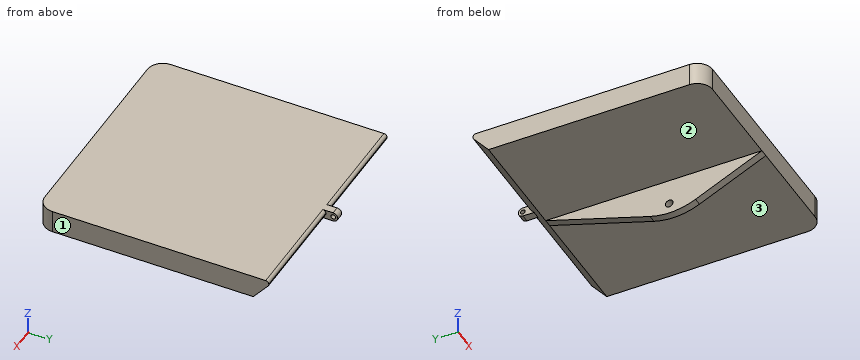
```python
from build123d import *

# Parameters (mm, degrees)
F0_W     = 150
F0_H     = 15
F1_DEPTH = 75
F2_SIZE2 = 10.0691955741
F2_SIZE  = 12
F3_R     = 2
F4_R     = 2.5
F5_DEPTH = 2.5
F6_R     = 1.5
F7_DEPTH = 2.5
F8_R     = 10


with BuildPart() as f1:
    # F0 (on Right) → F1 (new body, symmetric)
    with BuildSketch(Plane.YZ):
        with Locations((15, 24.5)):
            Rectangle(F0_W, F0_H)
    extrude(amount=F1_DEPTH, both=True)

    # F2
    f2_edges = [f1.edges().sort_by_distance(p)[0] for p in [
        (0, 90, 17),
    ]]
    f2_side = f1.faces().sort_by_distance((0, 90, 24.5))[0]
    chamfer(f2_edges, length=F2_SIZE, length2=F2_SIZE2, reference=f2_side)

    # F3
    f3_edges = [f1.edges().sort_by_distance(p)[0] for p in [
        (0, 90, 32),
        (0, 90, 29),
    ]]
    fillet(f3_edges, radius=F3_R)

    # F4 (on Right) → F5 (join, symmetric)
    with BuildSketch(Plane.YZ):
        with BuildLine():
            Line((79.9308044259, 17), (-60, 17))
            Line((-60, 17), (-17.0128849215, -3.2016815445))
            ThreePointArc((-17.0128849215, -3.2016815445), (-2.4781851934, -6.9231586695), (12.4051748829, -5.0277745355))
            Line((12.4051748829, -5.0277745355), (79.9308044259, 17))
        make_face()
        Circle(F4_R, mode=Mode.SUBTRACT)
    extrude(amount=F5_DEPTH, both=True)

    # F6 (on Right) → F7 (join, symmetric)
    with BuildSketch(Plane.YZ):
        with BuildLine():
            Line((94.6649461985, 32), (84.0871334076, 32))
            Line((84.0871334076, 32), (84.0871334076, 26))
            Line((84.0871334076, 26), (94.6649461985, 26))
            ThreePointArc((94.6649461985, 26), (97.6649461985, 29), (94.6649461985, 32))
        make_face()
        with Locations((94.6649461985, 29)):
            Circle(F6_R, mode=Mode.SUBTRACT)
    extrude(amount=F7_DEPTH, both=True)

    # F8
    f8_edges = [f1.edges().sort_by_distance(p)[0] for p in [
        (75, -60, 24.5),
        (-75, -60, 24.5),
    ]]
    fillet(f8_edges, radius=F8_R)


solid = f1.part
```
The listing builds one solid part. Answer for the finished solid, in the listing's coordinates (mm). Face numbers are marked on the shaded views. A direction names the side the tool comes from. Give positions to 0.01 mm unless a question says otherwise; leave off trailing zeros. Order: outer loops, then holes, each group sorted by start corner. A loop starts at its lowest first (then second) coordinate and runs counter-clockwise, first axis right, second up. Notation, with made-up numbers: M 88,-27.5 L 119,-27.5 A19 ccw 119,-3.5 Z; hole C 56.5,-11.75 d6. An arc over 180 degrees is marked long. Put each result on its own line as item: value. Start each with the question number.
Item 1: The part is cut by section D-D, the plane x = 37.5. Determine the outline of the cut face in (y, z).
Item 2: Which of the six approach directions +Z, -Z, +X, -X, +Y, -Y give full straight-line access (tool end or side, diameter ignored) to the marked faces 1, 2 and 3?
Item 3: The part is cut by section B-B, the plane y = 0. Determine the outline of the cut face in (x, z), and give its area (4 significant figures).
Item 4: Find the intervals of material crossed by line 1 along Z through (x, y) = (1, 0); line 2 along Z through (x, y) = (24, -2.5); line 3 along X through (y, z) = (-43.5, 10.5), in increasing order.
Item 5: The part is cut by section C-C, the plane z = 0. Determine the outline of the cut face in (x, y).
Item 6: The part is cut by section A-A, the plane x = 0.5. Determine the outline of the cut face in (y, z), and give its area (3 significant figures).
Item 7: Flat-ended cylindrical pins translate along their axes: P1, Ø10, axis at y = -39, z = 3, coming from the -X side; P2, Ø10, axis at x = 35.5, y = 8, coming from the -Z side; P3, Ø3.5, axis at y = 94.66, z = 29, coming from the +X side. Find the tip coordinate at first contact, or state that the pin passes through.
Answer key:
1. outline: M -60,17 L 79.93,17 L 89.53,28.44 A2 ccw 90,29.73 L 90,30 A2 ccw 88,32 L -60,32 Z
2. face 1: +Z, -Z, +X, +Y, -Y
2. face 2: -Z, -X, +Y, -Y
2. face 3: -Z, +X, +Y, -Y
3. outline: M -75,17 L -2.5,17 L -2.5,2.5 L 2.5,2.5 L 2.5,17 L 75,17 L 75,32 L -75,32 Z; M -2.5,-7 L 2.5,-7 L 2.5,-2.5 L -2.5,-2.5 Z
3. area: 2,345 mm²
4. line 1: z = -7 to -2.5, 2.5 to 32
4. line 2: z = 17 to 32
4. line 3: x = -2.5 to 2.5
5. outline: M -2.5,-23.83 L 2.5,-23.83 L 2.5,-2.5 L -2.5,-2.5 Z; M -2.5,2.5 L 2.5,2.5 L 2.5,27.82 L -2.5,27.82 Z
6. outline: M -60,17 L -17.01,-3.2 A40 ccw 12.41,-5.03 L 79.93,17 L 87.48,26 L 94.66,26 A3 ccw 94.66,32 L -60,32 Z; hole C 0,0 d5; hole C 94.66,29 d3
6. area: 4,060 mm²
7. P1: stops at x = -2.5
7. P2: stops at z = 17
7. P3: stops at x = 2.5
